Geometry check sheet. Reference: drawing and pictorial views, mm from the part's lowest x, y, z. A direction names the side the tool comes from. Round coordinates to 2 decimals unless told otherwise and drop trailing zeros. Order: outer loops, then holes, each group sorted by start corner. A loop starts at its lowest first (then second) coordinate and runs counter-clockwise, first axis right, second up.
Q1. Cross-section at D-D on y = 183. Record the cut outline in (x, z).
Q2. Set-up check for the marked faces 1, 2 and 3: record each of +Z, -Z, +X, -X, +Y, -Y from which the full face is reachable in a straight line by a thin tool's end or side.
Q3. Scan lines: probe 1 along X at (y, z) = (340, 103.5); probe 2 along Y at (x, z) = (75.5, 44); probe 3 along Y at (x, z) = (531, 186). Record each from-to range of solid material in increasing order.
Q4. Depth check by flat-ended pin: P1, Ø12, axis at x = 579, z = 670, coming from the +Y side; P2, Ø1, axis at x = 206, z = 873.5, coming from the -Y side; P3, Ø5, axis at y = 956.5, z = 344, coming from the -X side. Enter the tip coordinate at first touch or a pass-through.
Q5. Mould release check, pull along X, two halves, no side actions. Record for the marked faces 4, 5 and 6: +X half, -X half, draft (parallel to the pull), parting line (faces both ways), or undercut.
Q6. Cross-section at A-A on y = 857.5. Record the cut outline in (x, z).
Q7. Cross-section at B-B on z = 485. Record the cut outline in (x, y), then the cut area to 3 significant figures.
Q8. Cross-section at C-C on x = 481. Record the cut outline in (y, z), then the cut area to 3 significant figures.
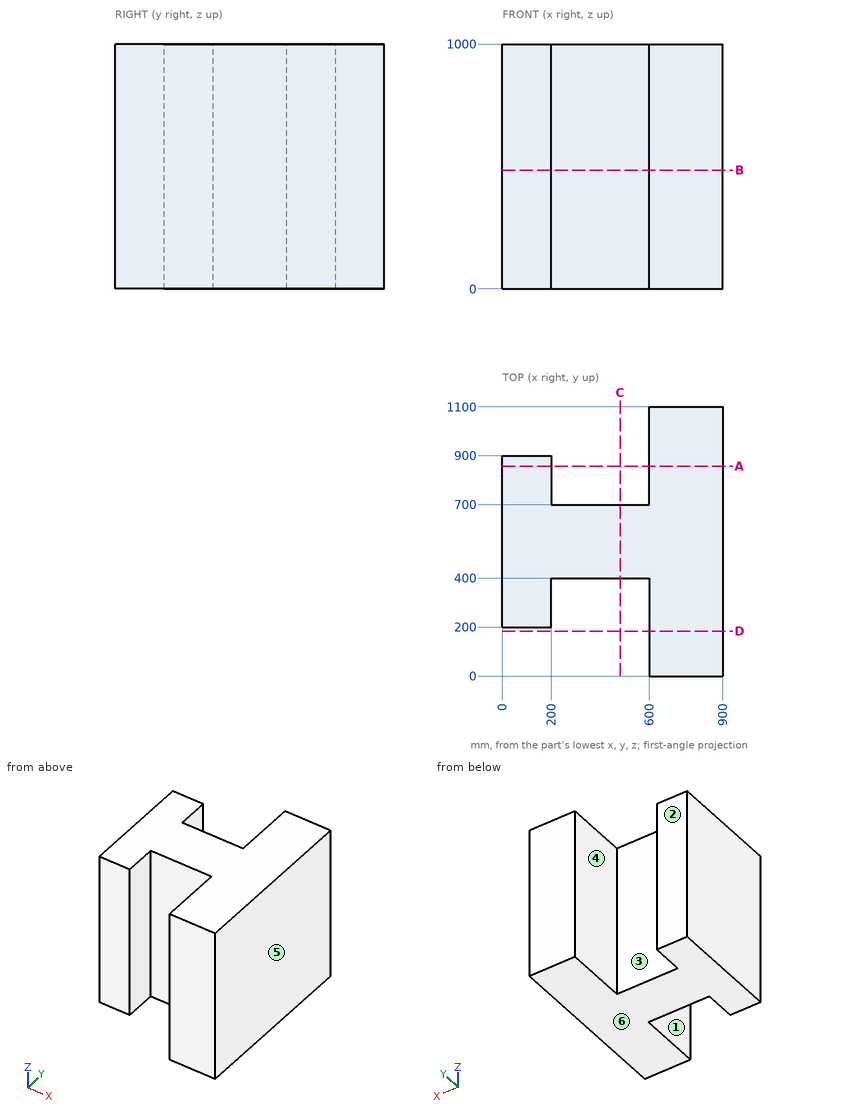
Results found:
1. outline: (600, 0) - (900, 0) - (900, 1000) - (600, 1000) - close
2. face 1: +Z, -Z, -Y
2. face 2: +Z, -Z, -X, +Y
2. face 3: +Z, -Z, +Y
3. probe 1: x = 0 to 200, 600 to 900
3. probe 2: y = 200 to 900
3. probe 3: y = 400 to 700
4. P1: stops at y = 700
4. P2: stops at y = 400
4. P3: stops at x = 600
5. face 4: undercut
5. face 5: +X half
5. face 6: draft
6. outline: (0, 0) - (200, 0) - (200, 1000) - (0, 1000) - close; (600, 0) - (900, 0) - (900, 1000) - (600, 1000) - close
7. outline: (0, 200) - (200, 200) - (200, 400) - (600, 400) - (600, 0) - (900, 0) - (900, 1100) - (600, 1100) - (600, 700) - (200, 700) - (200, 900) - (0, 900) - close
7. area: 590,000 mm2
8. outline: (400, 0) - (700, 0) - (700, 1000) - (400, 1000) - close
8. area: 300,000 mm2
